Can you work these out from the model? Positions are in its coordinate system, mm. Face numbers are marked on the shaded views. A direction names the side the tool comes from. Give positions to 0.01 mm unless a question says otherwise; leave off trailing zeros. Loops run counter-clockwise (first coordinate to the right, second up) from the corner with the lowest first, then second, coordinate; pieces in that order, holes last. Notation, with made-up numbers: (61, 56.5) - (96, 56.5) arc R30 ccw to (96, 89.5) - close; hole circle Ø5 at (1.5, 75.25). An arc over 180 degrees is marked (long way). Answer in a Markdown table with one row per item.
from build123d import *

# Parameters (mm, degrees)
BOSS_EXTRUDE1_DEPTH = 5.08
BOSS_EXTRUDE2_DEPTH = 61.595
BOSS_EXTRUDE3_DEPTH = 5.08
SKETCH4_R           = 3.302
CUT_EXTRUDE1_DEPTH  = 150.974308337
SKETCH5_R           = 2.667
CUT_EXTRUDE2_DEPTH  = 5.08


with BuildPart() as part:
    # Sketch1 → Boss-Extrude1 (new body)
    with BuildSketch(Plane(origin=(0, 0, 0), x_dir=(1, 0, 0), z_dir=(0, 1, 0))):
        Polygon((0, 64.005979691), (0, 43.18), (0, 0), (118.11, 0), (118.11, 43.18), align=None)
    extrude(amount=BOSS_EXTRUDE1_DEPTH)

    # Sketch2 → Boss-Extrude2 (add)
    with BuildSketch(Plane.XZ):
        Polygon((5.08, -5.08), (5.08, -57.951871441), (113.03, -38.917373874), (113.03, -5.08), (113.03, 0), (118.11, 0), (118.11, -43.18), (0, -64.005979691), (0, 0), (5.08, 0), align=None)
    extrude(amount=BOSS_EXTRUDE2_DEPTH)

    # Sketch3 → Boss-Extrude3 (add)
    with BuildSketch(Plane.XZ.offset(61.595)):
        Polygon((113.03, 0), (69.85, 0), (69.85, -31.75), (19.05, -31.75), (19.05, 0), (5.08, 0), (5.08, -57.951871441), (113.03, -38.917373874), align=None)
        Polygon((0, -64.005979691), (118.11, -43.18), (118.11, 0), (113.03, 0), (113.03, -38.917373874), (5.08, -57.951871441), (5.08, 0), (0, 0), align=None)
    extrude(amount=BOSS_EXTRUDE3_DEPTH)

    # Sketch4 → Cut-Extrude1 (cut, through all)
    with BuildSketch(Plane.ZY):
        with Locations((-12.7, -20.955)):
            Circle(SKETCH4_R)
        with Locations((-12.7, -40.005)):
            Circle(SKETCH4_R)
    extrude(amount=-CUT_EXTRUDE1_DEPTH, mode=Mode.SUBTRACT)

    # Sketch5 → Cut-Extrude2 (cut)
    with BuildSketch(Plane(origin=(10.945667174, 0, -62.075963247), x_dir=(-0.9848077530122081, 0, -0.17364817766693075), z_dir=(0.17364817766693075, 0, -0.9848077530122081))):
        with Locations(Location((-93.301496832, -6.985, 0), (0, 0, 180))):
            Circle(SKETCH5_R)
        with Locations((-93.301496832, -54.61)):
            Circle(SKETCH5_R)
        with Locations((-4.401496832, -6.985)):
            Circle(SKETCH5_R)
        with Locations(Location((-4.401496832, -54.61, 0), (0, 0, 180))):
            Circle(SKETCH5_R)
    extrude(amount=-CUT_EXTRUDE2_DEPTH, mode=Mode.SUBTRACT)


solid = part.part
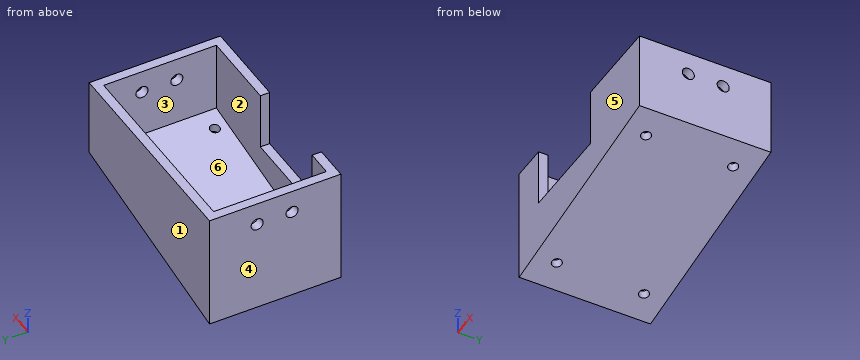
Q1. If I drill on line 1 (Y direction, x = 116.05, z = -12.7) (3 decimals); line 2 (Y direction, x = 94, z = -39) (3 decimals); line 3 (X direction, y = -36, z = -20.5), over which ranges is the centre line in solid material (lowest first)? Write a range as [from, to].
Checked values:
| item | result |
|---|---|
| line 1 | y = [-66.675, -43.307], [-36.703, -24.257], [-17.653, 5.08] |
| line 2 | y = [-66.675, -61.595], [0, 5.08] |
| line 3 | x = [0, 5.08], [113.03, 118.11] |
Q2. Imagine slicing it at C-C, the plane x = 68.5. Write out the boundary of the cut face in (y, z) (3 decimals), and give its area (3 significant figures).
Checked values:
| item | result |
|---|---|
| outline | (-66.675, -51.928) - (5.08, -51.928) - (5.08, 0) - (0, 0) - (0, -46.769) - (-61.595, -46.769) - (-61.595, -31.75) - (-66.675, -31.75) - close |
| area | 684 mm² |
Q3. For pin 1 (4 mm diameter, centred on y = -65, z = -15.5, fed in from -X); pin 2 (1.5 mm diameter, centred on x = 50, y = -65.5, fed in from +Z); pin 3 (12 mm diameter, centred on x = 69.5, y = -6.5, fed in from +Z); pin 4 (6 mm diameter, centred on x = 82.5, y = -26.5, fed in from +Z), each with a flat end and sliding along its axis, tell me the tip position at first contact or that it passes through.
Checked values:
| item | result |
|---|---|
| pin 1 | stops at x = 0 |
| pin 2 | stops at z = -31.75 |
| pin 3 | stops at z = -45.53 |
| pin 4 | stops at z = -43.77 |
Q4. Imagine slicing it at A-A, the plane z = -12.7. Write out the boundary of the cut face in (x, y) (3 decimals).
Checked values:
| item | result |
|---|---|
| outline | (0, -66.675) - (19.05, -66.675) - (19.05, -61.595) - (5.08, -61.595) - (5.08, -43.307) - (0, -43.307) - close; (0, -36.703) - (5.08, -36.703) - (5.08, -24.257) - (0, -24.257) - close; (0, -17.653) - (5.08, -17.653) - (5.08, 0) - (113.03, 0) - (113.03, -17.653) - (118.11, -17.653) - (118.11, 5.08) - (0, 5.08) - close; (69.85, -66.675) - (118.11, -66.675) - (118.11, -43.307) - (113.03, -43.307) - (113.03, -61.595) - (69.85, -61.595) - close; (113.03, -36.703) - (118.11, -36.703) - (118.11, -24.257) - (113.03, -24.257) - close |
Q5. On a 3-axis mill with a long thin cutter (end or side, diameter ignored), from which of +Z, -Z, +X, -X, +Y, -Y can I reach the whole of each face in a straight line? I mean the marked faces 1 and 2. Say none if no direction works.
Checked values:
| item | result |
|---|---|
| face 1 | +Z, -Z, +X, -X, +Y |
| face 2 | +Z |
Q6. If we mould it in two halves opening along X, with no side actions, what happens to the marked faces 3, 4, 5 and 6? For each: released by +X, released by -X, zero draft, split by the parting line, or undercut.
Checked values:
| item | result |
|---|---|
| face 3 | undercut |
| face 4 | released by -X |
| face 5 | zero draft |
| face 6 | undercut |
Q7. Imagine slicing it at B-B, the plane y = -35. Write out the boundary of the cut face in (x, z).
Checked values:
| item | result |
|---|---|
| outline | (0, -64.01) - (118.11, -43.18) - (118.11, 0) - (113.03, 0) - (113.03, -38.92) - (5.08, -57.95) - (5.08, 0) - (0, 0) - close |
